Input: part model. Units: mm. Frame: model coordinates. A direction names the side the tool comes from. Give positions to 0.01 mm unless a question says otherwise; leave off trailing zeros. Loops run counter-clockwise (first coordinate to the right, second up) from the corner with the lowest first, then second, coordinate; pieces in that order, holes last. Notation, with made-up numbers: (71.5, 77) - (106.5, 77) arc R35 ccw to (106.5, 115) - close; hole circle Ø3 at (-39, 70). An arc over 180 degrees is marked (long way). Answer as a JSON object with one key per item and string values.
from build123d import *

# Parameters (mm, degrees)
SKETCH1_W                          = 42.3
SKETCH1_H                          = 42.3
BOSS_EXTRUDE1_DEPTH                = 33
SKETCH2_R                          = 2.5
BOSS_EXTRUDE3_DEPTH                = 18
HOLE_FOR_M3_300_SC_NUTS_SP_2_D     = 4.22
HOLE_FOR_M3_300_SC_NUTS_SP_2_DEPTH = 4.5
HOLE_FOR_M3_300_SC_NUTS_SP_2_TIP   = 1.267815906
SKETCH5_R                          = 11
BOSS_EXTRUDE4_DEPTH                = 2


with BuildPart() as part:
    # Sketch1 → Boss-Extrude1 (new body)
    with BuildSketch(Plane(origin=(0, 0, 0), x_dir=(1, 0, 0), z_dir=(0, 1, 0))):
        with Locations((21.15, 21.15)):
            Rectangle(SKETCH1_W, SKETCH1_H)
    extrude(amount=BOSS_EXTRUDE1_DEPTH)

    # Sketch2 → Boss-Extrude3 (add)
    with BuildSketch(Plane(origin=(0, 0, 0), x_dir=(-1, 0, 0), z_dir=(0, -1, 0))):
        with Locations(Location((-21.15, 21.15, 0), (0, 0, 270))):
            Circle(SKETCH2_R)
    extrude(amount=BOSS_EXTRUDE3_DEPTH)

    # Hole for M3 300® SC Nuts (SP)2
    with Locations(Plane(origin=(0, 0, 0), x_dir=(-1, 0, 0), z_dir=(0, -1, 0))):
        with Locations((-5.65, 36.65), (-5.65, 5.65), (-36.65, 5.65), (-36.65, 36.65)):
            Hole(HOLE_FOR_M3_300_SC_NUTS_SP_2_D / 2, depth=HOLE_FOR_M3_300_SC_NUTS_SP_2_DEPTH)
            with Locations((0, 0, -(HOLE_FOR_M3_300_SC_NUTS_SP_2_DEPTH + HOLE_FOR_M3_300_SC_NUTS_SP_2_TIP / 2))):  # 118° drill point
                Cone(0, HOLE_FOR_M3_300_SC_NUTS_SP_2_D / 2, HOLE_FOR_M3_300_SC_NUTS_SP_2_TIP, mode=Mode.SUBTRACT)

    # Sketch5 → Boss-Extrude4 (add)
    with BuildSketch(Plane(origin=(0, 0, 0), x_dir=(1, 0, 0), z_dir=(0, 1, 0))):
        with Locations(Location((21.15, 21.15, 0), (0, 0, 270))):
            Circle(SKETCH5_R)
    extrude(amount=-BOSS_EXTRUDE4_DEPTH)


solid = part.part
Item 1: Material intervals for line 1 (Z direction, x = 5.65, y = 1.4); line 2 (X direction, y = 1.65, z = -36.65); line 3 (Z direction, x = 5, y = 2), sorted ascending. Write a range as [from, to].
Geometry check:
{"line 1": "z = [-42.3, -38.76], [-34.54, -7.76], [-3.54, 0]", "line 2": "x = [0, 3.54], [7.76, 34.54], [38.76, 42.3]", "line 3": "z = [-42.3, -38.66], [-34.64, -7.66], [-3.64, 0]"}
Item 2: Mould query, pull axis X, two halves, no side actions, for faces 3 (the face through (42.3, 16, -21)), 4 (the face through (21.04, -9.888, -23.648)), 5 (the face through (21, 16, 0)), 6 (the face through (38.6, 2.28, -35.84)). Classes: released by +X, released by -X, zero draft, split by the parting line, or undercut.
Geometry check:
{"face 3": "released by +X", "face 4": "split by the parting line", "face 5": "zero draft", "face 6": "undercut"}
Item 3: Contact query for flat-ended pins moving along their axis: P1, Ø4, axis at x = 36.65, z = -36.65, coming from the -Y side; P2, Ø12, axis at x = 33.5, z = -35.5, coming from the -Y side; P3, Ø2.5, axis at x = 5.65, z = -5.65, coming from the -Y side; P4, Ø5, axis at y = -3.5, z = -5.5, coming from the -X side. Output: stop coordinate, or through.
Geometry check:
{"P1": "stops at y = 4.57", "P2": "stops at y = 0", "P3": "stops at y = 5.02", "P4": "passes through"}
Item 4: Cut plane C-C (z = -21.15). Return loops of the section in (x, y), then the cut area to 3 significant figures.
Geometry check:
{"outline": "(0, 0) - (10.15, 0) - (10.15, -2) - (18.65, -2) - (18.65, -18) - (23.65, -18) - (23.65, -2) - (32.15, -2) - (32.15, 0) - (42.3, 0) - (42.3, 33) - (0, 33) - close", "area": "1,520 mm2"}
Item 5: Cut plane A-A (y = 1.5). Return loops of the section in (x, z), then the cut area to 3 significant figures.
Geometry check:
{"outline": "(0, -42.3) - (42.3, -42.3) - (42.3, 0) - (0, 0) - close; hole circle Ø4.22 at (5.65, -36.65); hole circle Ø4.22 at (5.65, -5.65); hole circle Ø4.22 at (36.65, -36.65); hole circle Ø4.22 at (36.65, -5.65)", "area": "1,730 mm2"}
Item 6: Cut plane D-D (x = 28). Return loops of the section in (y, z), then the cut area to 3 significant figures.
Geometry check:
{"outline": "(-2, -29.76) - (0, -29.76) - (0, -42.3) - (33, -42.3) - (33, 0) - (0, 0) - (0, -12.54) - (-2, -12.54) - close", "area": "1,430 mm2"}
Item 7: Cut plane B-B (x = 21.15). Return loops of the section in (y, z).
Geometry check:
{"outline": "(-18, -23.65) - (-2, -23.65) - (-2, -32.15) - (0, -32.15) - (0, -42.3) - (33, -42.3) - (33, 0) - (0, 0) - (0, -10.15) - (-2, -10.15) - (-2, -18.65) - (-18, -18.65) - close"}
Item 8: Access query for faces 1 (the face through (6.624, 2.281, -34.778)), 2 (the face through (0, 16, -21)). Directions: +Z, -Z, +X, -X, +Y, -Y. A direction counts if a zero-diameter tool reaches every point of the face in a straight line with its end or side. Return the directions, or none.
Geometry check:
{"face 1": "-Y", "face 2": "+Z, -Z, -X, +Y, -Y"}
